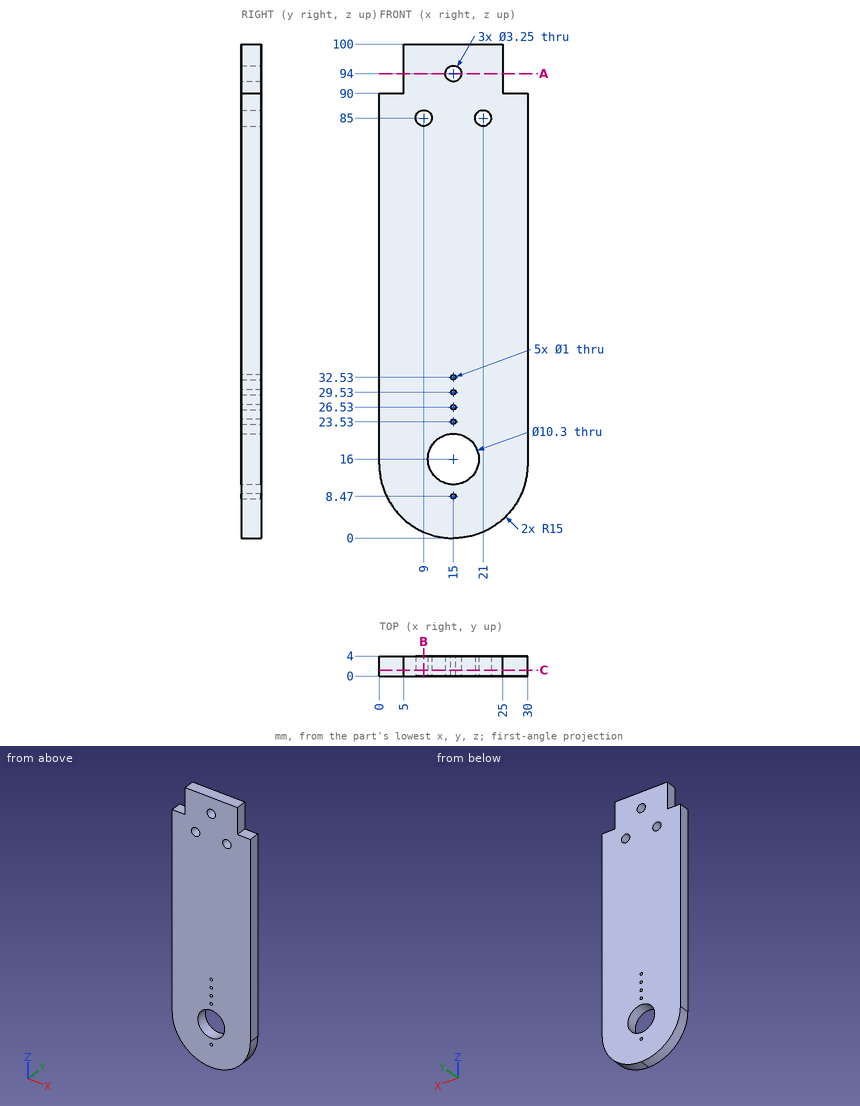
Geometry: see drawing. Coordinates: mm, zero at the bounding-box minimum. Give positions to 0.01 mm unless a question says otherwise; leave off trailing zeros. Loops run counter-clockwise (first coordinate to the right, second up) from the corner with the lowest first, then second, coordinate; pieces in that order, holes last. Notation, with made-up numbers: (5.25, -7.75) -> (44.25, -7.75) arc R17 cw to (44.25, 17.25) -> close; hole circle Ø5 at (74, 41). An arc over 180 degrees is marked (long way). Answer as a JSON object with one key per item and string values. Group by question number.
Item 1: Cut plane A-A, the plane z = 94. Return the cut outline in (x, y) (3 decimals), and give its area (3 significant figures).
Item 2: Line query: probe 1 along X at (y, z) = (2.1, 26.53); probe 2 along X at (y, z) = (1.6, 16); probe 3 along Z at (x, y) = (18.5, 2.1). Output: solid intervals per line, ascending.
Item 3: Pin query (flat end, axial travel): P1, Ø2, axis at y = 1.5, z = 95, coming from the -X side; P2, Ø2, axis at x = 7, y = 3, coming from the -Z side; P3, Ø2, axis at x = 28, y = 1, coming from the +Z side. Return the tip coordinate at first contact, or that it passes through.
Item 4: Cut plane B-B, the plane x = 9. Return the cut outline in (y, z) (3 decimals), and give its area (3 significant figures).
Item 5: Cut plane C-C, the plane y = 1.2. State how many separate pieces and enclosed holes the cut face has, and give its area (3 significant figures).
Checks:
{
 "1": {"outline": "(5, 0) -> (13.375, 0) -> (13.375, 4) -> (5, 4) -> close; (16.625, 0) -> (25, 0) -> (25, 4) -> (16.625, 4) -> close", "area": "67.0 mm²"},
 "2": {"probe 1": "x = 0 to 14.5, 15.5 to 30", "probe 2": "x = 0 to 9.85, 20.15 to 30", "probe 3": "z = 0.41 to 12.22, 19.78 to 100"},
 "3": {"P1": "stops at x = 5", "P2": "stops at z = 1.73", "P3": "stops at z = 90"},
 "4": {"outline": "(0, 1.252) -> (4, 1.252) -> (4, 83.375) -> (0, 83.375) -> close; (0, 86.625) -> (4, 86.625) -> (4, 100) -> (0, 100) -> close", "area": "382 mm²"},
 "5": {"separate pieces": "1", "enclosed holes": "9", "area": "2,690 mm²"}
}
